from build123d import *

# Parameters (mm, degrees)
BOSS_EXTRUDE1_DEPTH            = 5
BOSS_EXTRUDE1_DEPTH_BACK       = 5
F_4_0MM_DOWEL_HOLE2_AT_2_COUNT = 2
F_4_0MM_DOWEL_HOLE2_AT_2_PITCH = 20
FILLET1_R                      = 3
F_8_0MM_DOWEL_HOLE1_AT_2_COUNT = 2
F_8_0MM_DOWEL_HOLE1_AT_2_PITCH = 20


with BuildPart() as part:
    # Sketch1 → Boss-Extrude1 (new body, two sides)
    with BuildSketch(Plane.XY) as boss_extrude1_sk:
        with BuildLine():
            Line((-18, 0), (-5, 0))
            Line((-5, 0), (-5, 4))
            ThreePointArc((-5, 4), (0, 9), (5, 4))
            Line((5, 4), (5, 0))
            Line((5, 0), (22, 0))
            Line((22, 0), (22, 4))
            Line((22, 4), (8, 4))
            ThreePointArc((8, 4), (0, 12), (-8, 4))
            Line((-8, 4), (-18, 4))
            Line((-18, 4), (-18, 0))
        make_face()
    extrude(amount=BOSS_EXTRUDE1_DEPTH)
    extrude(boss_extrude1_sk.sketch, amount=-BOSS_EXTRUDE1_DEPTH_BACK)

    # Sketch7 → 4.0mm Dowel Hole2 (revolve, cut)
    with BuildSketch(Plane(origin=(10, 4, 0), x_dir=(0, 0, 1), z_dir=(1, 0, 0))):
        Polygon((0, 0), (0, 4), (2, 4), (2, 0.025), (2.025, 0), align=None)
    f_4_0mm_dowel_hole2 = revolve(axis=Axis((10, 10.35, 0), (0, -1, 0)), mode=Mode.SUBTRACT)

    # 4.0mm Dowel Hole2 at 2: 4.0mm Dowel Hole2 ×2
    with Locations(*[(-i * F_4_0MM_DOWEL_HOLE2_AT_2_PITCH, 0, 0) for i in range(1, F_4_0MM_DOWEL_HOLE2_AT_2_COUNT)]):
        add(f_4_0mm_dowel_hole2, mode=Mode.SUBTRACT)

    # Fillet1
    fillet1_edges = [part.edges().sort_by_distance(p)[0] for p in [
        (22, 2, -5),
        (-18, 2, 5),
        (22, 2, 5),
        (-18, 2, -5),
    ]]
    fillet(fillet1_edges, radius=FILLET1_R)

    # Sketch10 → 8.0mm Dowel Hole1 (revolve, cut)
    with BuildSketch(Plane(origin=(-10, 4, 0), x_dir=(0, 0, -1), z_dir=(1, 0, 0))):
        Polygon((0, 0), (0, 8), (4, 8), (4, 0.025), (4.025, 0), align=None)
    f_8_0mm_dowel_hole1 = revolve(axis=Axis((-10, -2.35, 0), (0, 1, 0)), mode=Mode.SUBTRACT)

    # 8.0mm Dowel Hole1 at 2: 8.0mm Dowel Hole1 ×2
    with Locations(*[(i * F_8_0MM_DOWEL_HOLE1_AT_2_PITCH, 0, 0) for i in range(1, F_8_0MM_DOWEL_HOLE1_AT_2_COUNT)]):
        add(f_8_0mm_dowel_hole1, mode=Mode.SUBTRACT)


solid = part.part
Source: CAD feature listing. Evaluate the final solid. Frame: model axes, mm. A direction names the side the tool comes from. Give positions to 0.01 mm unless a question says otherwise; leave off trailing zeros. Write each loop counter-clockwise with the first axis right and the second up, starting at its lowest first coordinate (ties: lowest second). Pieces come first, ordered by that corner, then holes. Notation, with made-up numbers: M 36.25,36.5 L 94.25,36.5 A16 ccw 94.25,67.5 Z; hole C 56.5,76 d3. An arc over 180 degrees is marked long. Return JSON: item names as keys, results as strings. Group by question number.
1) Material intervals for line 1 along X through (y, z) = (0.95, 0); line 2 along Z through (x, y) = (-10, 1.55); line 3 along Y through (x, z) = (-13, 1), sorted ascending. Write a range as [from, to].
2) Pin query (flat end, axial travel): P1, Ø2, axis at x = -9, z = -0.5, coming from the -Y side; P2, Ø5, axis at y = 10.5, z = -3.5, coming from the -X side; P3, Ø1, axis at y = 8, z = 0, coming from the +X side; P4, Ø3, axis at x = 11, z = 0.5, coming from the +Y side. Return the tip coordinate at first contact, or that it passes through.
3) Cut plane D-D, the plane y = 5. Output: boundary loops of the cut face in (x, z).
4) Pull-direction query (Z, two-part tool) for faces 1 (the face through (8, 2, 0)), 2 (the face through (-17.1, 1.97, -4.14)), 3 (the face through (21.1, 2.03, 4.14)); classes: pulls with the +Z half, pulls with the -Z half, needs draft (parallel to the pull), parting line crosses it, or undercut.
5) Cut plane B-B, the plane x = -10. Output: boundary loops of the cut face in (y, z) (3 decimals), plus the area to 3 significant figures.
6) Cut plane C-C, the plane z = 0. Give the number of separate pieces and of enclosed holes in the cut face, plus the area to 3 significant figures.
7) Cut plane A-A, the plane y = 1.5. Output: boundary loops of the cut face in (x, z).
8) Set-up query: faces 4 (the face through (-17.14, 1.97, 4.1)), 5 (the face through (6, 6, 0)), 6 (the face through (-5, 2, 0)), 7 (the face through (6, 5, 5)), 8 (the face through (-6, 6, 0)). Return all of +Z, -Z, +X, -X, +Y, -Y with unobstructed straight access to the full face (end or side cutting, diameter ignored); none if empty.
Recorded:
{
 "1": {"line 1": "x = [-18, -12], [-8, -5], [5, 8], [12, 22]", "line 2": "z = [-5, -2], [2, 5]", "line 3": "y = [0, 4]"},
 "2": {"P1": "stops at y = 0", "P2": "stops at x = -6.93", "P3": "stops at x = 6.03", "P4": "stops at y = 4"},
 "3": {"outline": "M -7.94,-5 L -4.9,-5 L -4.9,5 L -7.94,5 L -7.94,3.43 A4 cw -7.94,-3.43 Z; M 4.9,-5 L 7.94,-5 L 7.94,-3.43 A4 cw 7.94,3.43 L 7.94,5 L 4.9,5 Z"},
 "4": {"face 1": "undercut", "face 2": "pulls with the -Z half", "face 3": "pulls with the +Z half"},
 "5": {"outline": "M 0,-5 L 4,-5 L 4,-2.025 L 3.975,-2 L 0,-2 Z; M 0,2 L 3.975,2 L 4,2.025 L 4,5 L 0,5 Z", "area": "24.0 mm²"},
 "6": {"separate pieces": "3", "enclosed holes": "0", "area": "135 mm²"},
 "7": {"outline": "M -18,-2 A3 ccw -15,-5 L -5,-5 L -5,5 L -15,5 A3 ccw -18,2 Z; M 5,-5 L 19,-5 A3 ccw 22,-2 L 22,2 A3 ccw 19,5 L 5,5 Z; hole C -10,0 d4; hole C 10,0 d4"},
 "8": {"face 4": "+Z, -X, +Y, -Y", "face 5": "+X, +Y", "face 6": "+Z, -Z, -Y", "face 7": "+Z, +X, -X, +Y, -Y", "face 8": "-X, +Y"}
}
